from build123d import *

# Parameters (mm, degrees)
F2_W     = 32.767532
F2_H     = 10.747779
F3_DEPTH = 23
F4_W     = 55
F4_H     = 6
F5_DEPTH = 19.3
F6_R     = 12.5
F7_DEPTH = 1.5


with BuildPart() as f1:
    # F0 (on Right) → F1 (revolve)
    with BuildSketch(Plane.YZ):
        Polygon((30.937984, -25), (30.937984, 0), (-47.062016, 0), (-47.062016, -5), (-24.062016, -5), (-24.062016, -9), (12.937984, -9), (12.937984, -25), align=None)
    revolve(axis=Axis((0, -8.062016, 0), (0, -1, 0)))

    # F2 (on face) → F3 (cut, through all)
    with BuildSketch(Plane.XZ.offset(47.062016)):
        with Locations((-0.172598, 8.37389)):
            Rectangle(F2_W, F2_H)
    extrude(amount=-F3_DEPTH, mode=Mode.SUBTRACT)

    # F4 (on face) → F5 (cut)
    with BuildSketch(Plane(origin=(0, 30.937984, 0), x_dir=(-1, 0, 0), z_dir=(0, 1, 0))):
        Rectangle(F4_W, F4_H)
    extrude(amount=-F5_DEPTH, mode=Mode.SUBTRACT)

    # F6 (on face) → F7 (cut)
    with BuildSketch(Plane(origin=(0, 30.937984, 0), x_dir=(-1, 0, 0), z_dir=(0, 1, 0))):
        Circle(F6_R)
    extrude(amount=-F7_DEPTH, mode=Mode.SUBTRACT)


solid = f1.part
Input: part model. Units: mm. Frame: model coordinates. A direction names the side the tool comes from. Give positions to 0.01 mm unless a question says otherwise; leave off trailing zeros. Write each loop counter-clockwise with the first axis right and the second up, starting at its lowest first coordinate (ties: lowest second). Pieces come first, ordered by that corner, then holes. Notation, with made-up numbers: M 12,15 L 49,15 A21 cw 49,24 Z; hole C 41,36.25 d8. An arc over 180 degrees is marked long. Write item = value, one per line. Start each with the question number.
1) Draft query along X for faces 5 (the flat face through (0, 12.938, -14)), 6 (the cylindrical face through (0.2, 30.2, -12.5)), 7 (the flat face through (0, 29.438, -7)), 8 (the cylindrical face through (-0.508, 22.064, -24.995)). Return one class per face: +X half, -X half, draft (parallel to the pull), parting line (faces both ways), or undercut.
2) Material intervals for line 1 along Z through (x, y) = (0, -29.5); line 2 along Y through (x, z) = (-6, 14); line 3 along X through (y, z) = (-18, 0), sorted ascending. Write a range as [from, to].
3) First-contact query: pin 1 Ø9 at (x, y) = (2, -37) entering from +Z; pin 2 Ø1.5 at (x, y) = (5, -1) entering from +Z; pin 3 Ø24 at (x, z) = (7, 18) entering from -Y; pin 4 Ø10.5 at (x, z) = (2, 8.5) entering from +Y. Flat tips, straight axial feed; report the tip coordinate or a pass-through.
4) Reachability of faces 1 (the flat face through (0, 11.638, 0)), 2 (the flat face through (0, 29.438, 7)), 3 (the flat face through (0, -36, 3)), 4 (the flat face through (0, 12.938, 14)) from +Z, -Z, +X, -X, +Y, -Y: full face, straight path, thin tool, end or side. Return the list, or none.
5) Cut plane A-A on x = 14. Return the cut outline in (y, z).
6) Cut plane B-B on z = 0. Return the cut outline in (x, y).
7) Cut plane C-C on y = 26.5. Return the cut outline in (x, z).
8) Cut plane D-D on x = 0. Return the cut outline in (y, z).
Solved:
q1.face_5 = draft
q1.face_6 = undercut
q1.face_7 = undercut
q1.face_8 = parting line
q2.line_1 = [-5, 3]
q2.line_2 = [12.94, 30.94]
q2.line_3 = [-9, 9]
q3.pin_1 = 3
q3.pin_2 = 7.93
q3.pin_3 = -24.06
q3.pin_4 = 30.94
q4.face_1 = +X, -X, +Y
q4.face_2 = +Y
q4.face_3 = +Z, +X, -X, -Y
q4.face_4 = +Z, -Y
q5.outline = M 12.94,-20.71 L 30.94,-20.71 L 30.94,-3 L 12.94,-3 Z; M 12.94,3 L 30.94,3 L 30.94,20.71 L 12.94,20.71 Z
q6.outline = M -9,-24.06 L -5,-24.06 L -5,-47.06 L 5,-47.06 L 5,-24.06 L 9,-24.06 L 9,11.64 L -9,11.64 Z
q7.outline = M -24.82,-3 A25 ccw 24.82,-3 Z; M -24.82,3 L 24.82,3 A25 ccw Z
q8.outline = M -47.06,-5 L -24.06,-5 L -24.06,-9 L 12.94,-9 L 12.94,-25 L 30.94,-25 L 30.94,-12.5 L 29.44,-12.5 L 29.44,-3 L 11.64,-3 L 11.64,3 L 29.44,3 L 29.44,12.5 L 30.94,12.5 L 30.94,25 L 12.94,25 L 12.94,9 L -24.06,9 L -24.06,3 L -47.06,3 Z
